from build123d import *

# Parameters (mm, degrees)
SKETCH1_W                                         = 75
SKETCH1_H                                         = 75
SKETCH1_R                                         = 11
SKETCH1_R_2                                       = 5
SKETCH1_R_3                                       = 1.5
BOSS_EXTRUDE1_DEPTH                               = 5
SKETCH3_W                                         = 75
SKETCH3_H                                         = 5
BOSS_EXTRUDE2_DEPTH                               = 15
CSK_FOR_M2_5_FLAT_HEAD_MACHINE_SCREW1_D           = 2.9
CSK_FOR_M2_5_FLAT_HEAD_MACHINE_SCREW1_CSINK_D     = 5.5
CSK_FOR_M2_5_FLAT_HEAD_MACHINE_SCREW1_CSINK_ANGLE = 90


with BuildPart() as part:
    # Sketch1 → Boss-Extrude1 (new body)
    with BuildSketch(Plane.XY):
        with Locations((1.86226596, 7.507049672)):
            Rectangle(SKETCH1_W, SKETCH1_H)
        with Locations((1.86226596, 7.507049672)):
            Circle(SKETCH1_R, mode=Mode.SUBTRACT)
        with Locations((1.409145794, 25.001182464)):
            Circle(SKETCH1_R_2, mode=Mode.SUBTRACT)
        with Locations((-23.582472479, 24.353867941)):
            Circle(SKETCH1_R_3, mode=Mode.SUBTRACT)
        with Locations((26.400764067, 25.648496986)):
            Circle(SKETCH1_R_3, mode=Mode.SUBTRACT)
    extrude(amount=BOSS_EXTRUDE1_DEPTH)

    # Sketch3 → Boss-Extrude2 (add)
    with BuildSketch(Plane.XY.offset(5)):
        with Locations((1.86226596, 42.507049672)):
            Rectangle(SKETCH3_W, SKETCH3_H)
    extrude(amount=BOSS_EXTRUDE2_DEPTH)

    # CSK for M2.5 Flat Head Machine Screw1 (through all)
    with Locations(Plane(origin=(0, 40.007049672, 0), x_dir=(-1, 0, 0), z_dir=(0, -1, 0))):
        with Locations((-27.36226596, -12.5), (23.63773404, -12.5)):
            CounterSinkHole(CSK_FOR_M2_5_FLAT_HEAD_MACHINE_SCREW1_D / 2, CSK_FOR_M2_5_FLAT_HEAD_MACHINE_SCREW1_CSINK_D / 2, counter_sink_angle=CSK_FOR_M2_5_FLAT_HEAD_MACHINE_SCREW1_CSINK_ANGLE)


solid = part.part
The model under review builds one solid part; all positions refer to its coordinate system, in mm. A direction names the side the tool comes from. Coordinates: 2 decimals unless noted, no trailing zeros. Write each loop counter-clockwise with the first axis right and the second up, starting at its lowest first coordinate (ties: lowest second). Pieces come first, ordered by that corner, then holes. Notation, with made-up numbers: (37.25, 17) -> (64.25, 17) arc R13 ccw to (64.25, 37) -> close; hole circle Ø1 at (67.25, -38). An arc over 180 degrees is marked (long way). Answer in a Markdown table with one row per item.
1. We need section C-C, the plane x = 18. State the section outline as (y, z) points.
Answers below:
| item | result |
|---|---|
| outline | (-29.99, 0) -> (45.01, 0) -> (45.01, 20) -> (40.01, 20) -> (40.01, 5) -> (-29.99, 5) -> close |
2. Clearance check with flat-ended pins moving along their axes: pin 1 Ø5 at (x, z) = (21.5, 10.5) entering from -Y; pin 2 Ø4 at (x, z) = (-23.64, 12.5) entering from -Y. State where each tip first meets the part, or that it passes through.
Answers below:
| item | result |
|---|---|
| pin 1 | stops at y = 40.01 |
| pin 2 | stops at y = 40.75 |
3. For faces 1 (the flat face through (10, -2, 5)), 2 (the flat face through (-35.638, 12.9, 4.8)), list the 3-axis set-ups (+Z, -Z, +X, -X, +Y, -Y) from which the entire face can be reached by the end or side of a thin tool; tool diameter is ignored.
Answers below:
| item | result |
|---|---|
| face 1 | +Z, +X, -X, -Y |
| face 2 | +Z, -Z, -X, +Y, -Y |
4. We need section A-A, the plane z = 12.5. State the section outline as (x, y) points.
Answers below:
| item | result |
|---|---|
| outline | (-35.64, 40.01) -> (-26.39, 40.01) -> (-25.09, 41.31) -> (-25.09, 45.01) -> (-35.64, 45.01) -> close; (-22.19, 41.31) -> (-20.89, 40.01) -> (24.61, 40.01) -> (25.91, 41.31) -> (25.91, 45.01) -> (-22.19, 45.01) -> close; (28.81, 41.31) -> (30.11, 40.01) -> (39.36, 40.01) -> (39.36, 45.01) -> (28.81, 45.01) -> close |
5. We need section D-D, the plane x = -0.5. State the section outline as (y, z) points, and give its area (3 significant figures).
Answers below:
| item | result |
|---|---|
| outline | (-29.99, 0) -> (-3.24, 0) -> (-3.24, 5) -> (-29.99, 5) -> close; (18.25, 0) -> (20.38, 0) -> (20.38, 5) -> (18.25, 5) -> close; (29.62, 0) -> (45.01, 0) -> (45.01, 20) -> (40.01, 20) -> (40.01, 5) -> (29.62, 5) -> close |
| area | 296 mm^2 |
6. We need section B-B, the plane y = 15. State the section outline as (x, z) points.
Answers below:
| item | result |
|---|---|
| outline | (-35.64, 0) -> (-6.19, 0) -> (-6.19, 5) -> (-35.64, 5) -> close; (9.92, 0) -> (39.36, 0) -> (39.36, 5) -> (9.92, 5) -> close |
7. Wall thickness on probe 1 along X at (y, z) = (43.45, 12.5); probe 2 along X at (y, z) = (8, 3.25); probe 3 along Z at (x, y) = (-30.5, 31.5): over which ranges is each line inside the solid? List them lowest first. Write a range as [from, to].
Answers below:
| item | result |
|---|---|
| probe 1 | x = [-35.64, -25.09], [-22.19, 25.91], [28.81, 39.36] |
| probe 2 | x = [-35.64, -9.13], [12.85, 39.36] |
| probe 3 | z = [0, 5] |
8. Draft analysis for pull direction Y (two halves, no side actions). For faces 3 (the cylindrical face through (28.7, 43.18, 13.06)), 4 (the cylindrical face through (27.83, 26.1, 2.46)), 5 (the flat face through (1, -29.993, 2)), state which applies: +Y half, -Y half, draft (parallel to the pull), parting line (faces both ways), or undercut.
Answers below:
| item | result |
|---|---|
| face 3 | draft |
| face 4 | undercut |
| face 5 | -Y half |
